```python
from build123d import *

# Parameters (mm, degrees)
BOSS_EXTRUDE1_DEPTH                  = 342.9
BOSS_EXTRUDE1_DEPTH_BACK             = 342.9
SKETCH3_W                            = 38.1
SKETCH3_H                            = 25.4
SKETCH3_W_2                          = 31.75
SKETCH3_H_2                          = 19.05
F_1_4_0_25_DIAMETER_HOLE2_AT_2_COUNT = 2
F_1_4_0_25_DIAMETER_HOLE2_AT_2_PITCH = 25.4
F_1_4_0_25_DIAMETER_HOLE2_AT_3_COUNT = 2
F_1_4_0_25_DIAMETER_HOLE2_AT_3_PITCH = 661.111799988
F_1_4_0_25_DIAMETER_HOLE2_AT_4_COUNT = 2
F_1_4_0_25_DIAMETER_HOLE2_AT_4_PITCH = 50.8
F_1_4_0_25_DIAMETER_HOLE2_AT_5_COUNT = 2
F_1_4_0_25_DIAMETER_HOLE2_AT_5_PITCH = 635.711799988
F_1_4_0_25_DIAMETER_HOLE3_D          = 6.35
F_5_32_0_15625_DIAMETER_HOLE1_D      = 3.96875
F_10_0_1935_DIAMETER_HOLE1_D         = 4.9149


with BuildPart() as part:
    # Sketch3 → Boss-Extrude1 (new, two sides: drawn at the far end of the back side and taken through both)
    with BuildSketch(Plane.XY.offset(-BOSS_EXTRUDE1_DEPTH_BACK)):
        Rectangle(SKETCH3_W, SKETCH3_H)
        Rectangle(SKETCH3_W_2, SKETCH3_H_2, mode=Mode.SUBTRACT)
    extrude(amount=BOSS_EXTRUDE1_DEPTH + BOSS_EXTRUDE1_DEPTH_BACK)

    # Sketch8 → 1/4 (0.25) Diameter Hole2 (revolve, cut)
    with BuildSketch(Plane(origin=(-19.05, 0, -330.2), x_dir=(0, 0, 1), z_dir=(0, 1, 0))):
        Polygon((0, 0), (0, 38.1), (3.9624, 38.1), (3.175, 37.194199916), (3.175, 0), align=None)
    f_1_4_0_25_diameter_hole2 = revolve(axis=Axis((-25.4, 0, -330.2), (1, 0, 0)), mode=Mode.SUBTRACT)

    # 1/4 (0.25) Diameter Hole2 at 2: 1/4 (0.25) Diameter Hole2 ×2
    with Locations(*[(0, 0, i * F_1_4_0_25_DIAMETER_HOLE2_AT_2_PITCH) for i in range(1, F_1_4_0_25_DIAMETER_HOLE2_AT_2_COUNT)]):
        add(f_1_4_0_25_diameter_hole2, mode=Mode.SUBTRACT)

    # 1/4 (0.25) Diameter Hole2 at 3: 1/4 (0.25) Diameter Hole2 ×2
    with Locations(*[(0, 0, i * F_1_4_0_25_DIAMETER_HOLE2_AT_3_PITCH) for i in range(1, F_1_4_0_25_DIAMETER_HOLE2_AT_3_COUNT)]):
        add(f_1_4_0_25_diameter_hole2, mode=Mode.SUBTRACT)

    # 1/4 (0.25) Diameter Hole2 at 4: 1/4 (0.25) Diameter Hole2 ×2
    with Locations(*[(0, 0, i * F_1_4_0_25_DIAMETER_HOLE2_AT_4_PITCH) for i in range(1, F_1_4_0_25_DIAMETER_HOLE2_AT_4_COUNT)]):
        add(f_1_4_0_25_diameter_hole2, mode=Mode.SUBTRACT)

    # 1/4 (0.25) Diameter Hole2 at 5: 1/4 (0.25) Diameter Hole2 ×2
    with Locations(*[(0, 0, i * F_1_4_0_25_DIAMETER_HOLE2_AT_5_PITCH) for i in range(1, F_1_4_0_25_DIAMETER_HOLE2_AT_5_COUNT)]):
        add(f_1_4_0_25_diameter_hole2, mode=Mode.SUBTRACT)

    # 1/4 (0.25) Diameter Hole3 (through all)
    with Locations(Plane(origin=(19.05, 0, 0), x_dir=(0, 0, -1), z_dir=(1, 0, 0))):
        with Locations((-280.111799988, 0), (-254.711799988, 0), (-229.311799988, 0), (254, 0), (228.6, 0), (203.2, 0)):
            Hole(F_1_4_0_25_DIAMETER_HOLE3_D / 2)

    # 5/32 (0.15625) Diameter Hole1 (through all)
    with Locations(Plane(origin=(19.05, 0, 0), x_dir=(0, 0, -1), z_dir=(1, 0, 0))):
        with Locations((152.4, 0), (-178.511799988, 0)):
            Hole(F_5_32_0_15625_DIAMETER_HOLE1_D / 2)

    # #10 (0.1935) Diameter Hole1 (through all)
    with Locations(Plane.ZY.offset(19.05)):
        with Locations((-184.15, 0), (210.261799988, 0)):
            Hole(F_10_0_1935_DIAMETER_HOLE1_D / 2)


solid = part.part
```
Source: CAD feature listing. Evaluate the final solid. Frame: model axes, mm. A direction names the side the tool comes from. Give positions to 0.01 mm unless a question says otherwise; leave off trailing zeros. Loops run counter-clockwise (first coordinate to the right, second up) from the corner with the lowest first, then second, coordinate; pieces in that order, holes last. Notation, with made-up numbers: (71.25, -8.5) -> (125.25, -8.5) arc R14 ccw to (125.25, -2.5) -> close; hole circle Ø2 at (15, 55.25). An arc over 180 degrees is marked (long way). Use a Markdown table: item, result. Add a question column.
(1) Section query A-A (x = 6.5). Output: boundary loops of the cut face in (y, z) (3 decimals).
(2) Access query for faces 1 (the face through (-19.05, 0, -5)), 2 (the face through (0, 9.525, -5)). Directions: +Z, -Z, +X, -X, +Y, -Y. A direction counts if a zero-diameter tool reaches every point of the face in a straight line with its end or side. Return the directions, or none.
(3) Section query B-B (z = 171). Output: boundary loops of the cut face in (x, y) (3 decimals).
(4) Ray query, line 1 (X direction, y = 6, z = 22) (3 decimals); line 2 (Y direction, x = 18.1, z = -152.4); line 3 (Y direction, x = 16.65, z = -228.6) (3 decimals). Return the intervals inside material, ascending.
(5) Pull-direction query (X, two-part tool) for faces 3 (the face through (0, 12.7, -5)), 4 (the face through (19.05, 0, -5)), 5 (the face through (-15.875, 0, -5)), 6 (the face through (0, -9.525, -5)); classes: +X half, -X half, draft (parallel to the pull), parting line (faces both ways), or undercut.
Checked values:
| question | item | result |
|---|---|---|
| 1 | outline | (-12.7, -342.9) -> (-9.525, -342.9) -> (-9.525, 342.9) -> (-12.7, 342.9) -> close; (9.525, -342.9) -> (12.7, -342.9) -> (12.7, 342.9) -> (9.525, 342.9) -> close |
| 2 | face 1 | +Z, -Z, -X, +Y, -Y |
| 2 | face 2 | +Z, -Z |
| 3 | outline | (-19.05, -12.7) -> (19.05, -12.7) -> (19.05, 12.7) -> (-19.05, 12.7) -> close; hole (-15.875, -9.525) -> (15.875, -9.525) -> (15.875, 9.525) -> (-15.875, 9.525) -> close |
| 4 | line 1 | -19.05 to -15.875, 15.875 to 19.05 |
| 4 | line 2 | -12.7 to -1.98, 1.98 to 12.7 |
| 4 | line 3 | -12.7 to -3.175, 3.175 to 12.7 |
| 5 | face 3 | draft |
| 5 | face 4 | +X half |
| 5 | face 5 | undercut |
| 5 | face 6 | undercut |
